Geometry check sheet. Reference: the model listing, model coordinates, mm. A direction names the side the tool comes from. Round coordinates to 2 decimals unless told otherwise and drop trailing zeros. Write each loop counter-clockwise with the first axis right and the second up, starting at its lowest first coordinate (ties: lowest second). Pieces come first, ordered by that corner, then holes.
Item 1: Cross-section at D-D (x = 53). Enter the section's corners in (y, z).
Item 2: Cross-section at C-C (z = 11). Enter the section's corners in (x, y), then the cut area to 3 significant figures.
Item 3: Scan lines: probe 1 along Y at (x, z) = (60, 7.75); probe 2 along Y at (x, z) = (60, 2.8); probe 3 along Z at (x, y) = (58.75, 30.5). Record each from-to range of solid material in increasing order.
Item 4: Draft check along Y on faces 3 (the face through (45.86, 32.1, 2.43)), 4 (the face through (66.2, 19.95, 1.93)), 5 (the face through (55, 25, 15.8)). Enter one of: pulls with the +Y half, pulls with the -Y half, needs draft (parallel to the pull), parting line crosses it, or undercut.
Item 5: Cross-section at B-B (y = 18). Enter the section's corners in (x, z), then the cut area to 3 significant figures.
Item 6: Depth check by flat-ended pin: P1, Ø5, axis at x = 51, y = 28, coming from the +Z side; P2, Ø2, axis at x = 50.5, z = 11.5, coming from the -Y side; P3, Ø4, axis at y = 12, z = 12, coming from the -X side. Enter the tip coordinate at first touch or a pass-through.
Item 7: Cross-section at A-A (x = 60). Enter the section's corners in (y, z), then the cut area to 3 significant figures.
Item 8: Access from +Z, -Z, +X, -X, +Y, -Y to the whole of each face (thin tool, end or side, straight path). Record for faces 1 (the face through (58.91, 26.33, 9.88)), 2 (the face through (74.1, 3.86, 2.43)).
from build123d import *

# Parameters (mm, degrees)
SKETCH006_W     = 30
SKETCH006_H     = 30
PAD003_DEPTH    = 4.8
SKETCH007_R     = 10.5
PAD004_DEPTH    = 11
SKETCH008_R     = 8.4
POCKET003_DEPTH = 12
SKETCH011_R     = 6.5
POCKET004_DEPTH = 3.801
FILLET002_R     = 3


with BuildPart() as part:
    # Sketch006 → Pad003 (new body)
    with BuildSketch(Plane.XY):
        Rectangle(SKETCH006_W, SKETCH006_H)
    extrude(amount=PAD003_DEPTH)

    # Sketch007 (on Face6 of Pad003) → Pad004 (join)
    with BuildSketch(Plane.XY.offset(4.8)):
        Circle(SKETCH007_R)
    extrude(amount=PAD004_DEPTH)

    # Sketch008 (on Face8 of Pad004) → Pocket003 (cut)
    with BuildSketch(Plane.XY.offset(15.8)):
        Circle(SKETCH008_R)
    extrude(amount=-POCKET003_DEPTH, mode=Mode.SUBTRACT)

    # Sketch011 (on Face10 of Pocket003) → Pocket004 (cut, through all)
    with BuildSketch(Plane.XY.offset(3.8)):
        Circle(SKETCH011_R)
    extrude(amount=-POCKET004_DEPTH, mode=Mode.SUBTRACT)

    # Fillet002
    fillet002_edges = [part.edges().sort_by_distance(p)[0] for p in [
        (15, -15, 2.4),
        (-15, -15, 2.4),
        (15, 15, 2.4),
        (-15, 15, 2.4),
    ]]
    fillet(fillet002_edges, radius=FILLET002_R)


with BuildPart() as part_1:
    # Body003 placement: moved
    add(part.part.moved(Location((60, 18, 0))))


solid = part_1.part
Resolved:
1. outline: (3, 0) - (33, 0) - (33, 4.8) - (25.83, 4.8) - (25.83, 15.8) - (22.64, 15.8) - (22.64, 3.8) - (13.36, 3.8) - (13.36, 15.8) - (10.17, 15.8) - (10.17, 4.8) - (3, 4.8) - close
2. outline: circle Ø21 at (60, 18); hole circle Ø16.8 at (60, 18)
2. area: 125 mm2
3. probe 1: y = 7.5 to 9.6, 26.4 to 28.5
3. probe 2: y = 3 to 11.5, 24.5 to 33
3. probe 3: z = 0 to 4.8
4. face 3: pulls with the +Y half
4. face 4: undercut
4. face 5: needs draft
5. outline: (45, 0) - (53.5, 0) - (53.5, 3.8) - (51.6, 3.8) - (51.6, 15.8) - (49.5, 15.8) - (49.5, 4.8) - (45, 4.8) - close; (66.5, 0) - (75, 0) - (75, 4.8) - (70.5, 4.8) - (70.5, 15.8) - (68.4, 15.8) - (68.4, 3.8) - (66.5, 3.8) - close
5. area: 124 mm2
6. P1: stops at z = 4.8
6. P2: stops at y = 11.84
6. P3: stops at x = 50.29
7. outline: (3, 0) - (11.5, 0) - (11.5, 3.8) - (9.6, 3.8) - (9.6, 15.8) - (7.5, 15.8) - (7.5, 4.8) - (3, 4.8) - close; (24.5, 0) - (33, 0) - (33, 4.8) - (28.5, 4.8) - (28.5, 15.8) - (26.4, 15.8) - (26.4, 3.8) - (24.5, 3.8) - close
7. area: 124 mm2
8. face 1: +Z
8. face 2: +Z, -Z, +X, -Y
